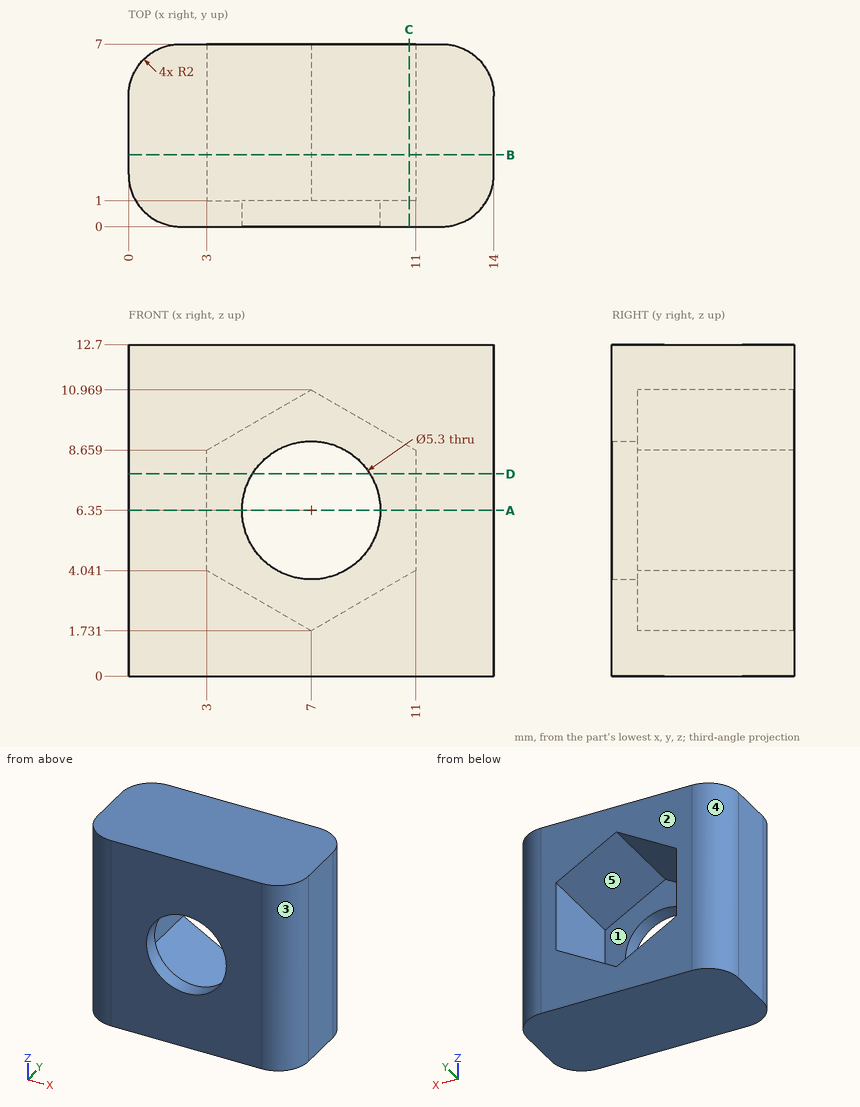
Input: dimensioned drawing with shaded views. Units: mm. Origin: part minimum x, y, z. A direction names the side the tool comes from. Round coordinates to 2 decimals unless told otherwise and drop trailing zeros. Loops run counter-clockwise (first coordinate to the right, second up) from the corner with the lowest first, then second, coordinate; pieces in that order, holes last. Notation, with made-up numbers: (50, -22.5) -> (77, -22.5) arc R23 ccw to (77, -13.5) -> close; hole circle Ø6 at (-23, -19.5). An arc over 180 degrees is marked (long way). Answer as a JSON object with one key per item and string values. Group by question number.
1) Section query C-C on x = 10.75. Output: boundary loops of the cut face in (y, z).
2) Draft query along X for the marked faces 3, 4 and 5. Return one class per face: +X half, -X half, draft (parallel to the pull), parting line (faces both ways), or undercut.
3) Reachability of the marked faces 1 and 2 from +Z, -Z, +X, -X, +Y, -Y: full face, straight path, thin tool, end or side. Return the list, or none.
4) Section query A-A on z = 6.35. Output: boundary loops of the cut face in (x, y).
5) Pin query (flat end, axial travel): pin 1 (4 mm diameter, centred on x = 7, z = 6.35, fed in from -Y); pin 2 (4 mm diameter, centred on x = 7.5, z = 5.5, fed in from +Y). Return the tip coordinate at first contact, or that it passes through.
6) Section query D-D on z = 7.75. Output: boundary loops of the cut face in (x, y).
7) Ray query, L1, parallel to Z at x = 7, y = 0.5; L2, parallel to X at y = 3, z = 8; L3, parallel to Y at x = 8, z = 3.25. Return the intervals inside material, ascending.
8) Section query B-B on y = 2.75. Output: boundary loops of the cut face in (x, z).
Reply:
{
 "1": {"outline": "(0, 0) -> (7, 0) -> (7, 3.9) -> (1, 3.9) -> (1, 8.8) -> (7, 8.8) -> (7, 12.7) -> (0, 12.7) -> close"},
 "2": {"face 3": "+X half", "face 4": "-X half", "face 5": "undercut"},
 "3": {"face 1": "+Y", "face 2": "+Z, -Z, +X, -X, +Y"},
 "4": {"outline": "(0, 2) arc R2 ccw to (2, 0) -> (4.35, 0) -> (4.35, 1) -> (3, 1) -> (3, 7) -> (2, 7) arc R2 ccw to (0, 5) -> close; (9.65, 0) -> (12, 0) arc R2 ccw to (14, 2) -> (14, 5) arc R2 ccw to (12, 7) -> (11, 7) -> (11, 1) -> (9.65, 1) -> close"},
 "5": {"pin 1": "passes through", "pin 2": "stops at y = 1"},
 "6": {"outline": "(0, 2) arc R2 ccw to (2, 0) -> (4.75, 0) -> (4.75, 1) -> (3, 1) -> (3, 7) -> (2, 7) arc R2 ccw to (0, 5) -> close; (9.25, 0) -> (12, 0) arc R2 ccw to (14, 2) -> (14, 5) arc R2 ccw to (12, 7) -> (11, 7) -> (11, 1) -> (9.25, 1) -> close"},
 "7": {"L1": "z = 0 to 3.7, 9 to 12.7", "L2": "x = 0 to 3, 11 to 14", "L3": "y = 0 to 1"},
 "8": {"outline": "(0, 0) -> (14, 0) -> (14, 12.7) -> (0, 12.7) -> close; hole (3, 4.04) -> (7, 1.73) -> (11, 4.04) -> (11, 8.66) -> (7, 10.97) -> (3, 8.66) -> close"}
}
